Read the model definition and answer for the solid it produces. Units are mm, in the model's axes. Face numbers are marked on the shaded views. Give positions to 0.01 mm unless a question says otherwise; leave off trailing zeros. Order: outer loops, then holes, each group sorted by start corner. A loop starts at its lowest first (then second) coordinate and runs counter-clockwise, first axis right, second up. Notation, with made-up numbers: (87, 10.5) - (92, 10.5) arc R10 cw to (92, 23.5) - close; hole circle Ø5 at (8, 76.25). An arc over 180 degrees is marked (long way). Return JSON: item names as keys, results as strings.
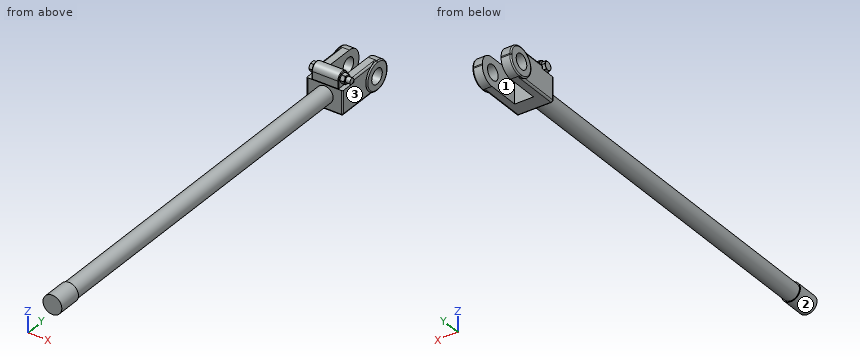
```python
from build123d import *

# Parameters (mm, degrees)
CROQUIS1_R              = 15.875
SALIENTE_EXTRUIR1_DEPTH = 40
CROQUIS2_R              = 14.2875
SALIENTE_EXTRUIR2_DEPTH = 615
CROQUIS3_W              = 65
CROQUIS3_H              = 48
SALIENTE_EXTRUIR3_DEPTH = 105
CROQUIS4_W              = 31.75
CROQUIS4_H              = 48
CORTAR_EXTRUIR1_DEPTH   = 78
REDONDEO1_R             = 23
CROQUIS5_R              = 12.7
CORTAR_EXTRUIR2_DEPTH   = 78
CORTAR_EXTRUIR3_DEPTH   = 2
CORTAR_EXTRUIR4_START   = -2
CORTAR_EXTRUIR4_DEPTH   = 2
REDONDEO3_R             = 3
REDONDEO4_START         = 654
REDONDEO4_DEPTH         = 56.5999999
REDONDEO4_START_2       = 710.5999999
REDONDEO4_2_DEPTH       = 24.0000002
REDONDEO4_START_3       = 27.4999999
REDONDEO4_3_DEPTH       = 3.0000001
REDONDEO4_START_4       = -30.5
REDONDEO4_4_DEPTH       = 3
REDONDEO5_R             = 2
REDONDEO6_R             = 2
CROQUIS9_W              = 7
CROQUIS9_H              = 24
CORTAR_EXTRUIR5_DEPTH   = 80
SALIENTE_EXTRUIR4_DEPTH = 53
REDONDEO7_R             = 3
CORTAR_EXTRUIR6_DEPTH   = 8
CROQUIS14_R             = 4.7625
CORTAR_EXTRUIR7_DEPTH   = 45
SALIENTE_EXTRUIR5_DEPTH = 7.5
CROQUIS16_R             = 6.71931732
CORTAR_EXTRUIR8_DEPTH   = 3
CORTAR_EXTRUIR8_DRAFT   = -64
REDONDEO8_R             = 1
CROQUIS17_R             = 4.7625
SALIENTE_EXTRUIR6_DEPTH = 60
CROQUIS18_R             = 4.7625
SALIENTE_EXTRUIR7_DEPTH = 7.5
CROQUIS19_R             = 6.761258256
CORTAR_EXTRUIR9_DEPTH   = 4
CORTAR_EXTRUIR9_DRAFT   = -52


with BuildPart() as part:
    # Croquis1 → Saliente-Extruir1 (new body)
    with BuildSketch(Plane(origin=(0, 0, 0), x_dir=(1, 0, 0), z_dir=(0, 1, 0))):
        with Locations(Location((0, 0, 0), (0, 0, 270))):
            Circle(CROQUIS1_R)
    extrude(amount=SALIENTE_EXTRUIR1_DEPTH)

    # Croquis2 → Saliente-Extruir2 (add)
    with BuildSketch(Plane(origin=(0, 40, 0), x_dir=(1, 0, 0), z_dir=(0, 1, 0))):
        with Locations(Location((0, 0, 0), (0, 0, 270))):
            Circle(CROQUIS2_R)
    extrude(amount=SALIENTE_EXTRUIR2_DEPTH)

    # Croquis3 → Saliente-Extruir3 (add)
    with BuildSketch(Plane(origin=(0, 655, 0), x_dir=(1, 0, 0), z_dir=(0, 1, 0))):
        Rectangle(CROQUIS3_W, CROQUIS3_H)
    extrude(amount=SALIENTE_EXTRUIR3_DEPTH)

    # Croquis4 → Cortar-Extruir1 (cut)
    with BuildSketch(Plane(origin=(0, 760, 0), x_dir=(1, 0, 0), z_dir=(0, 1, 0))):
        Rectangle(CROQUIS4_W, CROQUIS4_H)
    extrude(amount=-CORTAR_EXTRUIR1_DEPTH, mode=Mode.SUBTRACT)

    # Redondeo1
    redondeo1_edges = [part.edges().sort_by_distance(p)[0] for p in [
        (24.1875, 760, -24),
        (-24.1875, 760, 24),
        (-24.1875, 760, -24),
        (24.1875, 760, 24),
    ]]
    fillet(redondeo1_edges, radius=REDONDEO1_R)

    # Croquis5 → Cortar-Extruir2 (cut)
    with BuildSketch(Plane(origin=(32.5, 0, 0), x_dir=(0, 0, -1), z_dir=(1, 0, 0))):
        with Locations((0, 734.6)):
            Circle(CROQUIS5_R)
    extrude(amount=-CORTAR_EXTRUIR2_DEPTH, mode=Mode.SUBTRACT)

    # Croquis6 → Cortar-Extruir3 (cut)
    with BuildSketch(Plane(origin=(32.5, 0, 0), x_dir=(0, 0, -1), z_dir=(1, 0, 0))):
        with BuildLine():
            Line((24, 734.6), (24, 655))
            Line((24, 655), (-24, 655))
            Line((-24, 655), (-24, 734.6))
            ThreePointArc((-24, 734.6), (0, 710.6), (24, 734.6))
        make_face()
    extrude(amount=-CORTAR_EXTRUIR3_DEPTH, mode=Mode.SUBTRACT)

    # Croquis7 → Cortar-Extruir4 (cut)
    with BuildSketch(Plane.ZY.offset(32.5).offset(CORTAR_EXTRUIR4_START)):
        with BuildLine():
            Line((-24, 734.6), (-24, 655))
            Line((-24, 655), (24, 655))
            Line((24, 655), (24, 734.6))
            ThreePointArc((24, 734.6), (0, 710.6), (-24, 734.6))
        make_face()
    extrude(amount=CORTAR_EXTRUIR4_DEPTH, mode=Mode.SUBTRACT)

    # Redondeo3
    redondeo3_edges = [part.edges().sort_by_distance(p)[0] for p in [
        (30.5, 694.8, -24),
        (-30.5, 694.8, -24),
    ]]
    fillet(redondeo3_edges, radius=REDONDEO3_R)

    # Redondeo4: read off the stored shape, not the designer's step
    # Redondeo4 outline → Redondeo4 (cut)
    with BuildSketch(Plane(origin=(0, 0, 0), x_dir=(1, 0, 0), z_dir=(0, 1, 0)).offset(REDONDEO4_START)):
        with BuildLine():
            ThreePointArc((30.5, -21), (29.621320344, -23.121320344), (27.5, -24))
            Line((27.5, -24), (30.5, -24))
            Line((30.5, -24), (30.5, -21))
        make_face()
        with BuildLine():
            Line((-30.5, -24), (-27.5, -24))
            ThreePointArc((-27.5, -24), (-29.621320344, -23.121320344), (-30.5, -21))
            Line((-30.5, -21), (-30.5, -24))
        make_face()
    extrude(amount=REDONDEO4_DEPTH, mode=Mode.SUBTRACT)

    # Redondeo4 2 outline → Redondeo4 2 (cut)
    with BuildSketch(Plane(origin=(0, 0, 0), x_dir=(1, 0, 0), z_dir=(0, 1, 0)).offset(REDONDEO4_START_2)):
        with BuildLine():
            ThreePointArc((30.5, -21), (29.621320344, -23.121320344), (27.5, -24))
            Line((27.5, -24), (30.5, -24))
            Line((30.5, -24), (30.5, -21))
        make_face()
        with BuildLine():
            Line((-30.5, -24), (-27.5, -24))
            ThreePointArc((-27.5, -24), (-29.621320344, -23.121320344), (-30.5, -21))
            Line((-30.5, -21), (-30.5, -24))
        make_face()
    extrude(amount=REDONDEO4_2_DEPTH, mode=Mode.SUBTRACT)

    # Redondeo4 3 outline → Redondeo4 3 (add)
    with BuildSketch(Plane.YZ.offset(REDONDEO4_START_3)):
        with BuildLine():
            Line((734.6000001, 21), (734.6, 24))
            ThreePointArc((734.6, 24), (728.6, 23.237900077), (722.981049961, 21))
            Line((722.981049961, 21), (734.6000001, 21))
        make_face()
    extrude(amount=REDONDEO4_3_DEPTH)

    # Redondeo4 4 outline → Redondeo4 4 (add)
    with BuildSketch(Plane.YZ.offset(REDONDEO4_START_4)):
        with BuildLine():
            Line((734.6000001, 21), (734.6, 24))
            ThreePointArc((734.6, 24), (728.6, 23.237900077), (722.981049961, 21))
            Line((722.981049961, 21), (734.6000001, 21))
        make_face()
    extrude(amount=REDONDEO4_4_DEPTH)

    # Redondeo5
    redondeo5_edges = [part.edges().sort_by_distance(p)[0] for p in [
        (-32.5, 760, 0),
        (-32.5, 735.8, 24),
        (32.5, 735.8, 24),
        (-32.5, 735.8, -24),
        (-32.5, 753.263455967, -17.263455967),
        (-32.5, 753.263455967, 17.263455967),
        (32.5, 735.8, -24),
        (32.5, 760, 0),
        (32.5, 753.263455967, -17.263455967),
        (32.5, 753.263455967, 17.263455967),
        (32.5, 710.6, 0),
        (-32.5, 710.6, 0),
    ]]
    fillet(redondeo5_edges, radius=REDONDEO5_R - 0.0001)  # a hair under: the kernel refuses the full size

    # Redondeo6
    redondeo6_edges = [part.edges().sort_by_distance(p)[0] for p in [
        (-30.5, 655, 0),
        (0, 655, -24),
        (29.621320344, 655, -23.121320344),
        (-29.621320344, 655, -23.121320344),
        (30.5, 655, 0),
        (0, 655, 24),
        (-29.621320344, 655, 23.121320344),
        (29.621320344, 655, 23.121320344),
    ]]
    fillet(redondeo6_edges, radius=REDONDEO6_R)

    # Croquis9 → Cortar-Extruir5 (cut)
    with BuildSketch(Plane.ZY.offset(30.5)):
        with Locations((20.5, 667)):
            Rectangle(CROQUIS9_W, CROQUIS9_H)
    extrude(amount=-CORTAR_EXTRUIR5_DEPTH, mode=Mode.SUBTRACT)

    # Croquis10 → Saliente-Extruir4 (add)
    with BuildSketch(Plane.ZY.offset(30.5)):
        with BuildLine():
            Line((29.5, 678), (17, 678))
            Line((17, 678), (17, 656))
            Line((17, 656), (29.5, 656))
            ThreePointArc((29.5, 656), (40.5, 667), (29.5, 678))
        make_face()
    extrude(amount=-SALIENTE_EXTRUIR4_DEPTH)

    # Redondeo7
    redondeo7_edges = [part.edges().sort_by_distance(p)[0] for p in [
        (-29.621320344, 679, 23.121320344),
        (30.5, 679, 19),
        (29.621320344, 679, 23.121320344),
        (-30.5, 679, 19),
        (0, 679, 24),
    ]]
    fillet(redondeo7_edges, radius=REDONDEO7_R - 0.0001)  # a hair under: the kernel refuses the full size

    # Croquis11 → Cortar-Extruir6 (cut)
    with BuildSketch(Plane.ZY.offset(30.5)):
        with BuildLine():
            Line((29.5, 678), (17, 678))
            Line((17, 678), (17, 656))
            Line((17, 656), (29.5, 656))
            ThreePointArc((29.5, 656), (40.5, 667), (29.5, 678))
        make_face()
    extrude(amount=-CORTAR_EXTRUIR6_DEPTH, mode=Mode.SUBTRACT)

    # Croquis14 → Cortar-Extruir7 (cut)
    with BuildSketch(Plane.ZY.offset(22.5)):
        with Locations((29.5, 667)):
            Circle(CROQUIS14_R)
    extrude(amount=-CORTAR_EXTRUIR7_DEPTH, mode=Mode.SUBTRACT)

    # Croquis15 → Saliente-Extruir5 (add)
    with BuildSketch(Plane.ZY.offset(22.5)):
        Polygon((29.5, 659), (36.42820323, 663), (36.42820323, 671), (29.5, 675), (22.57179677, 671), (22.57179677, 663), align=None)
    extrude(amount=SALIENTE_EXTRUIR5_DEPTH)


with BuildPart() as cortar_extruir8_tool:
    # Croquis16 → Cortar-Extruir8 (with draft: the straight prism first)
    with BuildSketch(Plane.ZY.offset(30)):
        with BuildLine():
            Line((24.729588918, 691.570175939), (24.729588918, 678.749945473))
            Line((24.729588918, 678.749945473), (17.351920944, 678.749945473))
            Line((17.351920944, 678.749945473), (17.351920944, 645.064765076))
            ThreePointArc((17.351920944, 645.064765076), (54.036709128, 663.082957146), (24.729588918, 691.570175939))
        make_face()
        with Locations((29.345480417, 667)):
            Circle(CROQUIS16_R, mode=Mode.SUBTRACT)
    extrude(amount=-CORTAR_EXTRUIR8_DEPTH)
    # Cortar-Extruir8: the draft: its side faces are tilted about the plane it starts from
    cortar_extruir8_sides = [cortar_extruir8_tool.faces().sort_by_distance(p)[0] for p in [
        (-28.5, 685.160060706, 24.729588918),
        (-28.5, 678.749945473, 21.040754931),
        (-28.5, 661.907355274, 17.351920944),
        (-28.5, 663.082957146, 54.036709128),
        (-28.5, 667, 22.626163097),
    ]]
    draft(cortar_extruir8_sides, Plane.ZY.offset(30), CORTAR_EXTRUIR8_DRAFT)


with BuildPart() as part_1:
    add(part.part)

    # Cortar-Extruir8: cut by cortar_extruir8_tool
    add(cortar_extruir8_tool.part, mode=Mode.SUBTRACT)

    # Redondeo8
    redondeo8_edges = [part_1.edges().sort_by_distance(p)[0] for p in [
        (22.5, 667, 40.5),
        (22.5, 656, 23.25),
        (22.5, 678, 23.25),
        (-22.5, 667, 40.5),
        (-22.5, 656, 23.25),
        (-22.5, 678, 23.25),
    ]]
    fillet(redondeo8_edges, radius=REDONDEO8_R)

    # Croquis17 → Saliente-Extruir6 (add)
    with BuildSketch(Plane(origin=(-22.5, 0, 0), x_dir=(0, 0, -1), z_dir=(1, 0, 0))):
        with Locations(Location((-29.5, 667, 0), (0, 0, 180))):
            Circle(CROQUIS17_R)
    extrude(amount=SALIENTE_EXTRUIR6_DEPTH)

    # Croquis18 → Saliente-Extruir7 (add)
    with BuildSketch(Plane(origin=(22.5, 0, 0), x_dir=(0, 0, -1), z_dir=(1, 0, 0))):
        Polygon((-29.5, 675), (-36.42820323, 671), (-36.42820323, 663), (-29.5, 659), (-22.57179677, 663), (-22.57179677, 671), align=None)
        with Locations((-29.5, 667)):
            Circle(CROQUIS18_R, mode=Mode.SUBTRACT)
    extrude(amount=SALIENTE_EXTRUIR7_DEPTH)


with BuildPart() as cortar_extruir9_tool:
    # Croquis19 → Cortar-Extruir9 (with draft: the straight prism first)
    with BuildSketch(Plane(origin=(30, 0, 0), x_dir=(0, 0, -1), z_dir=(1, 0, 0))):
        with BuildLine():
            ThreePointArc((-24.252980935, 686.078510345), (-48.88237086, 663.019489242), (-17.15857321, 651.533586361))
            Line((-17.15857321, 651.533586361), (-17.15857321, 678.754417994))
            Line((-17.15857321, 678.754417994), (-24.252980935, 678.754417994))
            Line((-24.252980935, 678.754417994), (-24.252980935, 686.078510345))
        make_face()
        with Locations((-29.5, 667)):
            Circle(CROQUIS19_R, mode=Mode.SUBTRACT)
    extrude(amount=-CORTAR_EXTRUIR9_DEPTH)
    # Cortar-Extruir9: the draft: its side faces are tilted about the plane it starts from
    cortar_extruir9_sides = [cortar_extruir9_tool.faces().sort_by_distance(p)[0] for p in [
        (28, 665.144002178, 17.15857321),
        (28, 678.754417994, 20.705777072),
        (28, 682.41646417, 24.252980935),
        (28, 663.019489242, 48.88237086),
        (28, 667, 36.261258256),
    ]]
    draft(cortar_extruir9_sides, Plane(origin=(30, 0, 0), x_dir=(0, 0, -1), z_dir=(1, 0, 0)), CORTAR_EXTRUIR9_DRAFT)


with BuildPart() as part_2:
    add(part_1.part)

    # Cortar-Extruir9: cut by cortar_extruir9_tool
    add(cortar_extruir9_tool.part, mode=Mode.SUBTRACT)


solid = part_2.part
```
Q1. A cutting plane is placed at C-C (y = 122). Write down the section's boundary in (x, z) (1 decimal).
Values:
{"outline": "circle Ø28.6 at (0, 0)"}
Q2. Given pin 1 (10 mm diameter, centred on x = -4, z = 24.5, fed in from +Y); pin 2 (4 mm diameter, centred on y = 220, z = 13.5, fed in from -X); pin 3 (2 mm diameter, centred on x = -26, y = 665.5, fed in from +Z), each flat-ended and moving along its own axis, determine where each tip first touches the part or whether it passes through.
Values:
{"pin 1": "stops at y = 682", "pin 2": "stops at x = -8.48", "pin 3": "stops at z = 36.43"}
Q3. Determine the mould class of the marked faces 1, 2 and 3 for opening direction X: released by +X, released by -X, zero draft, split by the parting line, or undercut.
Values:
{"face 1": "undercut", "face 2": "split by the parting line", "face 3": "released by +X"}
Q4. Consider L1, parallel to Z at x = -20.75, y = 734.6; L2, parallel to X at y = 715.5, z = 6 (3 decimals); L3, parallel to Y at x = 20, z = 0. Determine where each line is inside the solid, lowest interval first.
Values:
{"L1": "z = -24 to -12.7, 12.7 to 24", "L2": "x = -32.5 to -15.875, 15.875 to 32.5", "L3": "y = 655 to 721.9, 747.3 to 760"}
Q5. A cutting plane is placed at A-A (y = 701). Write down the section's boundary in (x, z) (3 decimals).
Values:
{"outline": "(-30.5, -21) arc R3 ccw to (-27.5, -24) - (-15.875, -24) - (-15.875, 24) - (-27.5, 24) arc R3 ccw to (-30.5, 21) - close; (15.875, -24) - (27.5, -24) arc R3 ccw to (30.5, -21) - (30.5, 21) arc R3 ccw to (27.5, 24) - (15.875, 24) - close"}
